Verification items for the finished model (mm, model axes). Face numbers are marked on the shaded views. A direction names the side the tool comes from. Coordinates: 2 decimals unless noted, no trailing zeros. Order: outer loops, then holes, each group sorted by start corner. A loop starts at its lowest first (then second) coordinate and runs counter-clockwise, first axis right, second up. Notation, with made-up numbers: M -34.5,60 L -27.5,60 A11 cw -27.5,77 Z; hole C 50,-30.75 d9. An arc over 180 degrees is marked long. Return JSON: item names as keys, results as strings. Group by question number.
Q1. Section check D-D, the plane z = 2.9. Count the separate pieces of the cut face and the enclosed holes in it, then the cut area to 4 significant figures.
Q2. Thickness scan on probe 1 along Y at (x, z) = (7, 1.9); probe 2 along Y at (x, z) = (2, 0.3); probe 3 along X at (y, z) = (3, 0.85). Record the ranges inside material, lowest first.
Q3. Section check A-A, the plane x = 1.25. Enter the section's corners in (y, z), then the cut area to 3 significant figures.
Q4. Access from +Z, -Z, +X, -X, +Y, -Y to the whole of each face (thin tool, end or side, straight path). Record for the marked faces 1, 2 and 3.
Q5. Mould release check, pull along Y, two halves, no side actions. Record for the marked faces 4, 5 and 6: pulls with the +Y half, pulls with the -Y half, needs draft (parallel to the pull), parting line crosses it, or undercut.
Q6. Section check B-B, the plane y = -21.5. Enter the section's corners in (x, z), then the cut area to 4 significant figures.
Q7. Section check C-C, the plane x = 7.75. Enter the section's corners in (y, z).
Q8. Go/stop test with flat-tipped pins: pin 1 Ø1.6 at (y, z) = (16.5, 2.5) entering from +X; pin 2 Ø1.6 at (y, z) = (33.5, 1.5) entering from -X. Record where each tip stops, or that it passes through.
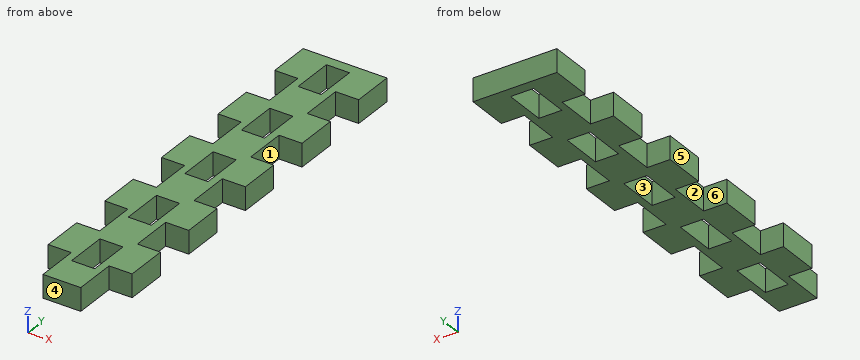
from build123d import *

# Parameters (mm, degrees)
SKETCH_1_W          = 20
SKETCH_1_H          = 100
EXTRUDE_1_DEPTH     = 5.5
SKETCH_2_W          = 5.5
SKETCH_2_H          = 10
CUT_EXTRUDE_1_DEPTH = 52.285962992
SKETCH_3_W          = 5.5
SKETCH_3_H          = 10
CUT_EXTRUDE_2_DEPTH = 52.285962992


with BuildPart() as part:
    # ｽｹｯﾁ1 → ﾎﾞｽ - 押し出し1 (new body)
    with BuildSketch(Plane.XY):
        Rectangle(SKETCH_1_W, SKETCH_1_H)
    extrude(amount=EXTRUDE_1_DEPTH)

    # ｽｹｯﾁ2 → ｶｯﾄ - 押し出し1 (cut, through all)
    with BuildSketch(Plane.XY.offset(5.5)):
        with Locations((-7.25, 35)):
            Rectangle(SKETCH_2_W, SKETCH_2_H)
        with Locations((-7.25, 15)):
            Rectangle(SKETCH_2_W, SKETCH_2_H)
        with Locations((-7.25, -5)):
            Rectangle(SKETCH_2_W, SKETCH_2_H)
        with Locations((-7.25, -25)):
            Rectangle(SKETCH_2_W, SKETCH_2_H)
        with Locations((7.25, -25)):
            Rectangle(SKETCH_2_W, SKETCH_2_H)
        with Locations((7.25, -5)):
            Rectangle(SKETCH_2_W, SKETCH_2_H)
        with Locations((7.25, 15)):
            Rectangle(SKETCH_2_W, SKETCH_2_H)
        with Locations((7.25, 35)):
            Rectangle(SKETCH_2_W, SKETCH_2_H)
        with Locations((-7.25, -45)):
            Rectangle(SKETCH_2_W, SKETCH_2_H)
        with Locations((7.25, -45)):
            Rectangle(SKETCH_2_W, SKETCH_2_H)
    extrude(amount=-CUT_EXTRUDE_1_DEPTH, mode=Mode.SUBTRACT)

    # ｽｹｯﾁ3 → ｶｯﾄ - 押し出し2 (cut, through all)
    with BuildSketch(Plane.XY.offset(5.5)):
        with Locations((0, -37.5)):
            Rectangle(SKETCH_3_W, SKETCH_3_H)
        with Locations((0, -17.5)):
            Rectangle(SKETCH_3_W, SKETCH_3_H)
        with Locations((0, 2.5)):
            Rectangle(SKETCH_3_W, SKETCH_3_H)
        with Locations((0, 22.5)):
            Rectangle(SKETCH_3_W, SKETCH_3_H)
        with Locations((0, 42.5)):
            Rectangle(SKETCH_3_W, SKETCH_3_H)
    extrude(amount=-CUT_EXTRUDE_2_DEPTH, mode=Mode.SUBTRACT)


solid = part.part
Numbers:
{
 "1": {"separate pieces": "1", "enclosed holes": "5", "area": "1,175 mm2"},
 "2": {"probe 1": "y = -40 to -30, -20 to -10, 0 to 10, 20 to 30, 40 to 50", "probe 2": "y = -50 to -42.5, -32.5 to -22.5, -12.5 to -2.5, 7.5 to 17.5, 27.5 to 37.5, 47.5 to 50", "probe 3": "x = -10 to -2.75, 2.75 to 10"},
 "3": {"outline": "M -50,0 L -42.5,0 L -42.5,5.5 L -50,5.5 Z; M -32.5,0 L -22.5,0 L -22.5,5.5 L -32.5,5.5 Z; M -12.5,0 L -2.5,0 L -2.5,5.5 L -12.5,5.5 Z; M 7.5,0 L 17.5,0 L 17.5,5.5 L 7.5,5.5 Z; M 27.5,0 L 37.5,0 L 37.5,5.5 L 27.5,5.5 Z; M 47.5,0 L 50,0 L 50,5.5 L 47.5,5.5 Z", "area": "275 mm2"},
 "4": {"face 1": "+Z, -Z, +X", "face 2": "+Z, -Z, -X", "face 3": "+Z, -Z"},
 "5": {"face 4": "pulls with the -Y half", "face 5": "needs draft", "face 6": "undercut"},
 "6": {"outline": "M -4.5,0 L -2.75,0 L -2.75,5.5 L -4.5,5.5 Z; M 2.75,0 L 4.5,0 L 4.5,5.5 L 2.75,5.5 Z", "area": "19.25 mm2"},
 "7": {"outline": "M -40,0 L -30,0 L -30,5.5 L -40,5.5 Z; M -20,0 L -10,0 L -10,5.5 L -20,5.5 Z; M 0,0 L 10,0 L 10,5.5 L 0,5.5 Z; M 20,0 L 30,0 L 30,5.5 L 20,5.5 Z; M 40,0 L 50,0 L 50,5.5 L 40,5.5 Z"},
 "8": {"pin 1": "stops at x = 4.5", "pin 2": "stops at x = -4.5"}
}
